Could you check a few things on this drawing? It's one solid part, dimensions in mm from its lowest x, y, z. A direction names the side the tool comes from. Round coordinates to 2 decimals unless told otherwise and drop trailing zeros. Loops run counter-clockwise (first coordinate to the right, second up) from the corner with the lowest first, then second, coordinate; pieces in that order, holes last. Notation, with made-up numbers: M -18.5,72.25 L 12.5,72.25 A27 ccw 12.5,88.25 Z; hole C 49.5,50 d11. An arc over 180 degrees is marked long. Write each question's results on one line, items separated by ' | '. Start each with the question number.
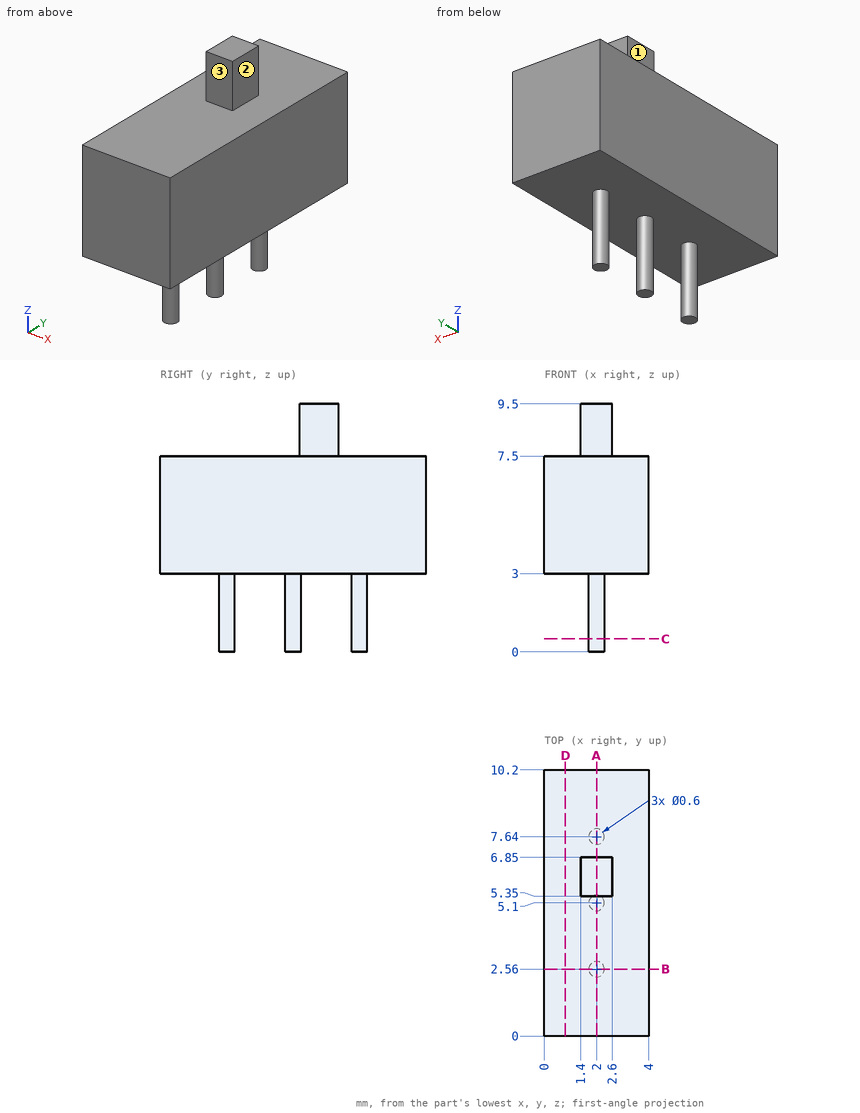
1. I want a section at A-A on x = 2. List the corners of the cut face in (y, z) for me, plus the area to 3 significant figures.
2. I want a section at B-B on y = 2.56. List the corners of the cut face in (x, z) for me.
3. I need wall thicknesses on line 1 along Y through (x, z) = (1.85, 0.75); line 2 along Z through (x, y) = (0.5, 1); line 3 along X through (y, z) = (6, 8.25). Which ranges of each line are inside material? Lowest first, please.
4. Which directions (+Z, -Z, +X, -X, +Y, -Y) give clear straight access to the entire face, cutting with the end or side of a thin tool? Please do the marked faces 1, 2 and 3.
5. I want a section at C-C on z = 0.5. List the corners of the cut face in (x, y) for me.
6. I want a section at D-D on x = 0.8. List the corners of the cut face in (y, z) for me, plus the area to 3 significant figures.
7. For pin 1 (1.2 mm diameter, centred on y = 6.5, z = 9, fed in from +X); pin 2 (0.6 mm diameter, centred on x = 2, z = 8.5, fed in from -Y); pin 3 (1 mm diameter, centred on x = 3.5, y = 3, fed in from +Z), each with a flat end and sliding along its axis, tell me the tip position at first contact or that it passes through.
Outcome:
1) outline: M 0,3 L 2.26,3 L 2.26,0 L 2.86,0 L 2.86,3 L 4.8,3 L 4.8,0 L 5.4,0 L 5.4,3 L 7.34,3 L 7.34,0 L 7.94,0 L 7.94,3 L 10.2,3 L 10.2,7.5 L 6.85,7.5 L 6.85,9.5 L 5.35,9.5 L 5.35,7.5 L 0,7.5 Z | area: 54.3 mm2
2) outline: M 0,3 L 1.7,3 L 1.7,0 L 2.3,0 L 2.3,3 L 4,3 L 4,7.5 L 0,7.5 Z
3) line 1: 2.3 to 2.82, 4.84 to 5.36, 7.38 to 7.9 | line 2: 3 to 7.5 | line 3: 1.4 to 2.6
4) face 1: +Z, -X, +Y, -Y | face 2: +Z, +X, +Y, -Y | face 3: +Z, +X, -X, -Y
5) outline: C 2,2.56 d0.6; C 2,5.1 d0.6; C 2,7.64 d0.6
6) outline: M 0,3 L 10.2,3 L 10.2,7.5 L 0,7.5 Z | area: 45.9 mm2
7) pin 1: x = 2.6 | pin 2: y = 5.35 | pin 3: z = 7.5
